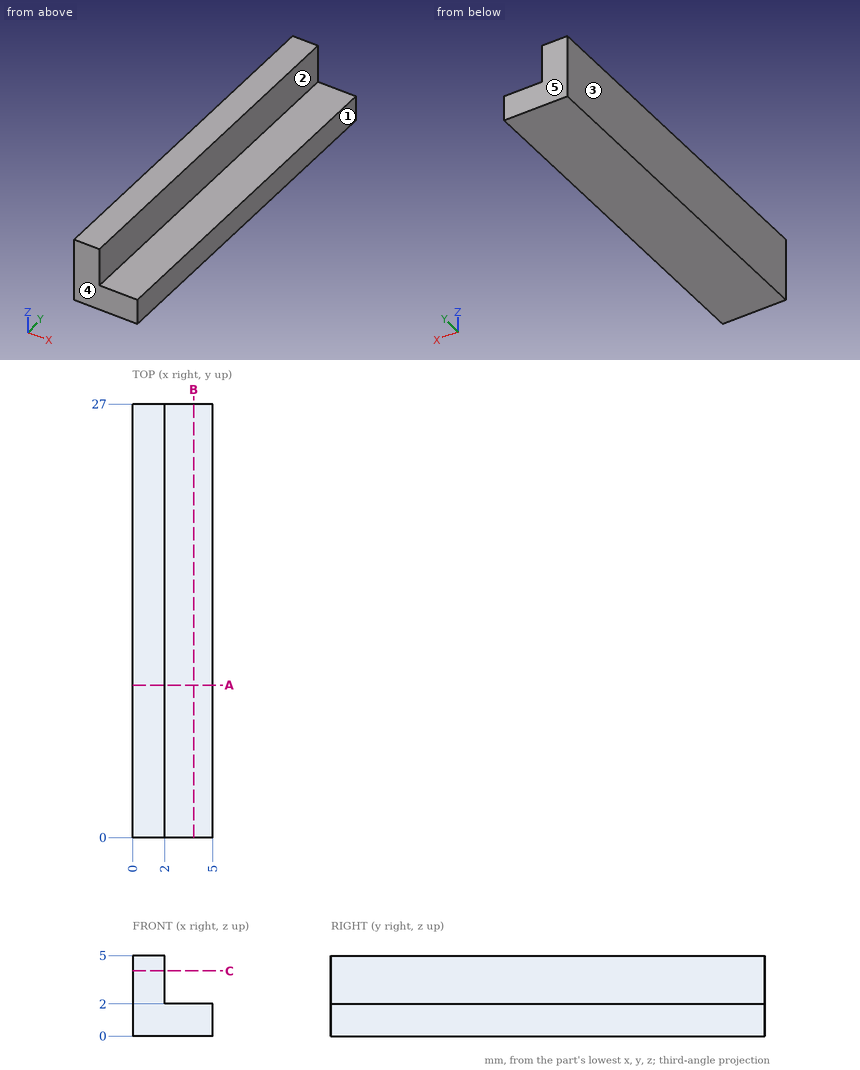
Geometry: see drawing. Coordinates: mm, zero at the bounding-box minimum. A direction names the side the tool comes from. Round coordinates to 2 decimals unless told otherwise and drop trailing zeros. Loops run counter-clockwise (first coordinate to the right, second up) from the corner with the lowest first, then second, coordinate; pieces in that order, holes last. Notation, with made-up numbers: M -30.5,74 L 1.5,74 A16 ccw 1.5,89 Z; hole C -37,35.25 d10. An arc over 180 degrees is marked long. Use a Markdown table: item, result. Add a question column.
1. Contact query for a flat-ended pin moving along its axis: pin 1 (2.5 mm diameter, centred on x = 3.5, y = 10.5, fed in from +Z). Output: stop coordinate, or through.
2. Cut plane C-C, the plane z = 4.05. Output: boundary loops of the cut face in (x, y), and give its area (3 significant figures).
3. Set-up query: the marked faces 1 and 2. Return all of +Z, -Z, +X, -X, +Y, -Y with unobstructed straight access to the full face (end or side cutting, diameter ignored); none if empty.
4. Cut plane A-A, the plane y = 9.5. Output: boundary loops of the cut face in (x, z).
5. Cut plane B-B, the plane x = 3.8. Output: boundary loops of the cut face in (y, z).
6. Ray query, line 1 along Z through (x, y) = (2.6, 10.5). Return the intervals inside material, ascending. Write a range as [from, to].
7. Pull-direction query (Y, two-part tool) for the marked faces 3, 4 and 5; classes: +Y half, -Y half, draft (parallel to the pull), parting line (faces both ways), or undercut.
Solution:
| question | item | result |
|---|---|---|
| 1 | pin 1 | stops at z = 2 |
| 2 | outline | M 0,0 L 2,0 L 2,27 L 0,27 Z |
| 2 | area | 54.0 mm2 |
| 3 | face 1 | +Z, -Z, +X, +Y, -Y |
| 3 | face 2 | +Z, +X, +Y, -Y |
| 4 | outline | M 0,0 L 5,0 L 5,2 L 2,2 L 2,5 L 0,5 Z |
| 5 | outline | M 0,0 L 27,0 L 27,2 L 0,2 Z |
| 6 | line 1 | z = [0, 2] |
| 7 | face 3 | draft |
| 7 | face 4 | -Y half |
| 7 | face 5 | +Y half |
